Build history of the part. All positions in model axes, mm. A direction names the side the tool comes from. Coordinates: 2 decimals unless noted, no trailing zeros. Loops run counter-clockwise (first coordinate to the right, second up) from the corner with the lowest first, then second, coordinate; pieces in that order, holes last. Notation, with made-up numbers: (76, 23) -> (95, 23) arc R19 cw to (95, 32) -> close; hole circle Ø1 at (47, -28). An arc over 180 degrees is marked (long way). One line per item, written item: value. Start each with the question number.
```python
from build123d import *

# Parameters (mm, degrees)
SKETCH1_R           = 5.08
BOSS_EXTRUDE1_DEPTH = 17.78
CUT_EXTRUDE1_DEPTH  = 15.24


with BuildPart() as part:
    # Sketch1 → Boss-Extrude1 (new body)
    with BuildSketch(Plane(origin=(0, 0, 0), x_dir=(1, 0, 0), z_dir=(0, 1, 0))):
        with BuildLine():
            Line((-32.154011799, -31.603429406), (-93.281689982, -28.139023899))
            Line((-93.281689982, -28.139023899), (-106.470617871, -7.793457389))
            Line((-106.470617871, -7.793457389), (-123.496324783, -7.793457389))
            Line((-123.496324783, -7.793457389), (-123.496324783, 1.798490167))
            Line((-123.496324783, 1.798490167), (-69.358514677, 22.660976101))
            Line((-69.358514677, 22.660976101), (-15.470629933, 42.347571766))
            ThreePointArc((-15.470629933, 42.347571766), (43.979702916, -9.921842389), (-32.154011799, -31.603429406))
        make_face()
        Circle(SKETCH1_R, mode=Mode.SUBTRACT)
    extrude(amount=BOSS_EXTRUDE1_DEPTH)

    # Sketch2 → Cut-Extrude1 (cut)
    with BuildSketch(Plane(origin=(0, 17.78, 0), x_dir=(1, 0, 0), z_dir=(0, 1, 0))):
        with BuildLine():
            Line((-14.599045148, 39.961793075), (-68.465982608, 20.282849978))
            Line((-68.465982608, 20.282849978), (-120.956324783, 0.055230443))
            Line((-120.956324783, 0.055230443), (-120.956324783, -5.253457389))
            Line((-120.956324783, -5.253457389), (-105.090165624, -5.253457389))
            Line((-105.090165624, -5.253457389), (-91.851329605, -25.676013414))
            Line((-91.851329605, -25.676013414), (-31.014061001, -29.123959985))
            ThreePointArc((-31.014061001, -29.123959985), (41.392622315, -9.835031413), (-14.599045148, 39.961793075))
        make_face()
    extrude(amount=-CUT_EXTRUDE1_DEPTH, mode=Mode.SUBTRACT)


solid = part.part
```
Item 1: Band-saw the part on B-B, the plane y = 8. List the corners of the cut face in (x, z) (1 decimal).
Item 2: Two-plate mould, pull along X, no slides. Class faces 3 (the face through (-0.661, 1.252, -5.037)), 4 (the face through (-115, 9, 7.793)), 5 (the face through (44.258, 8.766, 8.598)), 6 (the face through (-120.956, 10, 3)): +X half, -X half, draft (parallel to the pull), parting line (faces both ways), or undercut.
Item 3: Band-saw the part on C-C, the plane z = -25.5. List the corners of the cut face in (x, y).
Item 4: Drop flat-ended pins along their axis: pin 1 Ø5 at (x, z) = (-60, 2) entering from -Y; pin 2 Ø4 at (y, z) = (10, -12.5) entering from +X; pin 3 Ø4 at (x, y) = (-2.5, 9.5) entering from +Z; pin 4 Ø8 at (y, z) = (10.5, -33.5) entering from +X. Give the stop position or say it passes through.
Item 5: Band-saw the part on D-D, the plane x = 21.5. List the corners of the cut face in (y, z).
Item 6: Tool access for faces 1 (the face through (-98.563, 10.267, 15.322)), 2 (the face through (-62.29, 8.766, 29.895)): list every direction of +Z, -Z, +X, -X, +Y, -Y with a clear straight run to the whole face (end or side of a thin tool).
Item 7: Band-saw the part on A-A, the plane x = 0. List the corners of the cut face in (y, z) (3 decimals), and give its area (3 significant figures).
Item 8: Probe probe 1 along Z at (x, y) = (0, 1.9) (3 decimals); probe 2 along Z at (x, y) = (0, 14.5) (3 decimals); probe 3 along X at (y, z) = (0.85, 0) (3 decimals). List the from-to ranges inside material, lowest first.
Worked out:
1. outline: (-123.5, -1.8) -> (-69.4, -22.7) -> (-15.5, -42.3) arc R45.1 ccw (long way) to (-32.2, 31.6) -> (-93.3, 28.1) -> (-106.5, 7.8) -> (-123.5, 7.8) -> close; hole (-121, -0.1) -> (-68.5, -20.3) -> (-14.6, -40) arc R42.5 ccw (long way) to (-31, 29.1) -> (-91.9, 25.7) -> (-105.1, 5.3) -> (-121, 5.3) -> close
2. face 3: undercut
2. face 4: draft
2. face 5: parting line
2. face 6: undercut
3. outline: (-61.59, 0) -> (37.18, 0) -> (37.18, 17.78) -> (34.06, 17.78) -> (34.06, 2.54) -> (-54.19, 2.54) -> (-54.19, 17.78) -> (-61.59, 17.78) -> close
4. pin 1: stops at y = 0
4. pin 2: stops at x = 43.85
4. pin 3: stops at z = 45.08
4. pin 4: stops at x = 34.09
5. outline: (0, -39.63) -> (17.78, -39.63) -> (17.78, -36.71) -> (2.54, -36.71) -> (2.54, 36.71) -> (17.78, 36.71) -> (17.78, 39.63) -> (0, 39.63) -> close
6. face 1: +Y
6. face 2: +Z, -X, +Y, -Y
7. outline: (0, -45.085) -> (17.78, -45.085) -> (17.78, -42.545) -> (2.54, -42.545) -> (2.54, -5.08) -> (0, -5.08) -> close; (0, 5.08) -> (2.54, 5.08) -> (2.54, 42.545) -> (17.78, 42.545) -> (17.78, 45.085) -> (0, 45.085) -> close
7. area: 281 mm²
8. probe 1: z = -45.085 to -5.08, 5.08 to 45.085
8. probe 2: z = -45.085 to -42.545, 42.545 to 45.085
8. probe 3: x = -123.496 to -5.08, 5.08 to 45.085
